Part print with two shaded views. Sizes in mm from the minimum x, y, z corner. A direction names the side the tool comes from. Round coordinates to 2 decimals unless told otherwise and drop trailing zeros. Order: outer loops, then holes, each group sorted by start corner. A loop starts at its lowest first (then second) coordinate and runs counter-clockwise, first axis right, second up. Notation, with made-up numbers: (80, 34) - (100, 34) arc R13 cw to (100, 46) - close; hole circle Ø3 at (89.25, -30.75). An arc over 180 degrees is marked (long way). Write item = value, one per line.
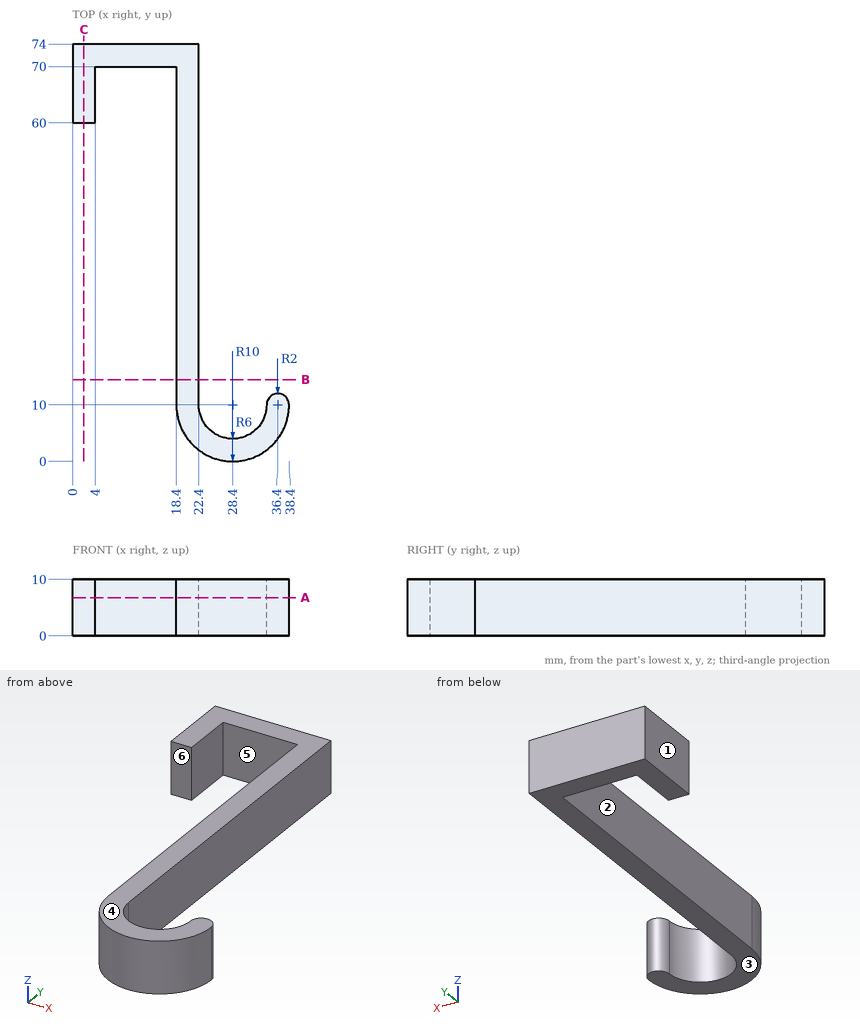
1) Flat gauge pins, fed straight in: pin 1 Ø4 at (x, z) = (21.5, 4.5) entering from -Y; pin 2 Ø1 at (x, z) = (25, 3.5) entering from -Y; pin 3 Ø1 at (y, z) = (26.5, 6) entering from +X; pin 4 Ø2 at (x, y) = (16.5, 35.5) entering from +Z. Where does each tip first touch, or does it go through?
Conclusion:
pin_1 = 1.28
pin_2 = 0.43
pin_3 = 22.4
pin_4 = through
2) Mould opens along X. For the marked faces 1, 2 and 3 say: +X half, -X half, draft (parallel to the pull), parting line (faces both ways), or undercut.
Conclusion:
face_1 = -X half
face_2 = undercut
face_3 = draft
3) 3-axis set-ups, long thin cutter, end or side, ignore diameter. For the marked faces 4, 5 and 6: which of +Z, -Z, +X, -X, +Y, -Y reach the whole face in a straight line?
Conclusion:
face_4 = +Z, +X, -X, +Y, -Y
face_5 = +Z, -Z, -Y
face_6 = +Z, -Z, -X, -Y
4) Cut at A-A (z = 6.75). Write the cut outline in (x, y), and give its area (3 significant figures).
Conclusion:
outline = (0, 60) - (4, 60) - (4, 70) - (18.4, 70) - (18.4, 10) arc R10 ccw to (38.4, 10) arc R2 ccw to (34.4, 10) arc R6 cw to (22.4, 10) - (22.4, 74) - (0, 74) - close
area = 476 mm^2
5) Cut at C-C (x = 2). Write the cut outline in (y, z).
Conclusion:
outline = (60, 0) - (74, 0) - (74, 10) - (60, 10) - close
6) Wall check: line 1 along X through (y, z) = (57, 1); line 2 along X through (y, z) = (10.5, 9.75); line 3 along X through (y, z) = (71, 3.5). Give the ranges that are in metal, low to high.
Conclusion:
line_1 = 18.4 to 22.4
line_2 = 18.4 to 22.4, 34.46 to 38.34
line_3 = 0 to 22.4
7) Cut at B-B (y = 14.5). Write the cut outline in (x, z), and give its area (3 significant figures).
Conclusion:
outline = (18.4, 0) - (22.4, 0) - (22.4, 10) - (18.4, 10) - close
area = 40.0 mm^2
